```python
from build123d import *

# Parameters (mm, degrees)
F1_DEPTH = 3
F2_R     = 1.25
F3_DEPTH = 12.5
F4_R     = 1.25
F5_DEPTH = 4


# Not quite as in the source:
# - a feature names something its author has since deleted; it is built from what else it names


with BuildPart() as f1:
    # F0 (on Top) → F1 (new body, symmetric)
    with BuildSketch(Plane.XY):
        Polygon((-38.3288674057, 0), (-57, 0), (-57, -2), (0, -2), (0, 0), (-3.9376540358, 0), (-6.9237630814, 0), (-9.9603020251, 0), (-9.9603020251, 3.6380901354), (-57.4212029734, 32.3077111831), (-58.4553107619, 30.595805496), (-38.3288674057, 18.4380610677), align=None)
        Polygon((-35.6059968472, 0), (-35.6059968472, 17.1079821885), (-12.5451418841, 3.3529622977), (-12.5451418841, 0), align=None, mode=Mode.SUBTRACT)
    extrude(amount=F1_DEPTH, both=True)

    # F2 (on face) → F3 (cut, symmetric)
    with BuildSketch(Plane.XZ.offset(2)):
        with Locations((-53, 0)):
            Circle(F2_R)
        with Locations((-4, 0)):
            Circle(F2_R)
    extrude(amount=F3_DEPTH, both=True, mode=Mode.SUBTRACT)

    # F4 (on face) → F5 (cut)
    with BuildSketch(Plane(origin=(-1.0527110533, -1.7427023171, 0), x_dir=(-0.8559528436, 0.5170538943, 0), z_dir=(0.5170538943, 0.8559528436, 0))):
        with Locations((63.8546698487, 0)):
            Circle(F4_R)
        with Locations((14.8546698487, 0)):
            Circle(F4_R)
    extrude(amount=-F5_DEPTH, mode=Mode.SUBTRACT)


solid = f1.part
```
Source: CAD feature listing. Evaluate the final solid. Frame: model axes, mm. A direction names the side the tool comes from. Coordinates: 2 decimals unless noted, no trailing zeros. Loops run counter-clockwise (first coordinate to the right, second up) from the corner with the lowest first, then second, coordinate; pieces in that order, holes last. Notation, with made-up numbers: M 16.25,44.5 L 28.25,44.5 A16 cw 28.25,62.5 Z; hole C 42,-17.75 d7. An arc over 180 degrees is marked long. Put each result on its own line as item: value. Start each with the question number.
1) Contact query for flat-ended pins moving along their axis: pin 1 Ø3 at (x, z) = (-26, -0.5) entering from +Y; pin 2 Ø1.6 at (y, z) = (-1.5, 0.5) entering from -X; pin 3 Ø3 at (y, z) = (2, 0.5) entering from +X; pin 4 Ø1.5 at (x, y) = (-13.5, 6) entering from +Z. Output: stop coordinate, or through.
2) Cut plane C-C on y = 7.5. Return the cut outline in (x, z), then the cut area to 3 significant figures.
3) Pull-direction query (X, two-part tool) for faces 4 (the face through (0, -1, 0)), 5 (the face through (-57.931, 31.464, 0.042)), 6 (the face through (-48, 0, 0)), 7 (the face through (-35.606, 8, 0)); classes: pulls with the +X half, pulls with the -X half, needs draft (parallel to the pull), parting line crosses it, or undercut.
4) Cut plane B-B on z = 2.4. Return the cut outline in (x, y).
5) Reachability of faces 1 (the face through (-12.545, 2, 0)), 2 (the face through (-48.53, 24.6, 0.04)), 3 (the face through (-51.81, -1.01, 0.38)) from +Z, -Z, +X, -X, +Y, -Y: full face, straight path, thin tool, end or side. Return the list, or none.
6) Cut plane A-A on x = -4. Return the cut outline in (y, z).
7) Cut plane D-D on x = -53. Return the cut outline in (y, z).
8) Ray query, L1, parallel to X at y = 1.5, z = -2.4; L2, parallel to Z at x = -53, y = -1.2; L3, parallel to Y at x = -18.5, z = 1.25. Return the intervals inside material, ascending. Write a range as from..to.
The answers:
1. pin 1: stops at y = 14.23
1. pin 2: stops at x = -57
1. pin 3: stops at x = -9.96
1. pin 4: stops at z = 3
2. outline: M -38.33,-3 L -35.61,-3 L -35.61,3 L -38.33,3 Z; M -19.5,-3 L -16.35,-3 L -16.35,3 L -19.5,3 Z
2. area: 35.2 mm²
3. face 4: pulls with the +X half
3. face 5: pulls with the -X half
3. face 6: needs draft
3. face 7: undercut
4. outline: M -58.46,30.6 L -38.33,18.44 L -38.33,0 L -57,0 L -57,-2 L 0,-2 L 0,0 L -9.96,0 L -9.96,3.64 L -57.42,32.31 Z; hole M -35.61,0 L -12.55,0 L -12.55,3.35 L -35.61,17.11 Z
5. face 1: +Z, -Z
5. face 2: +Z, -Z, -X
5. face 3: -Y
6. outline: M -2,-3 L 0,-3 L 0,-1.25 L -2,-1.25 Z; M -2,1.25 L 0,1.25 L 0,3 L -2,3 Z
7. outline: M -2,-3 L 0,-3 L 0,-1.25 L -2,-1.25 Z; M -2,1.25 L 0,1.25 L 0,3 L -2,3 Z; M 27.3,-3 L 29.64,-3 L 29.64,3 L 27.3,3 Z
8. L1: x = -38.33..-35.61, -12.55..-9.96
8. L2: z = -3..-1.25, 1.25..3
8. L3: y = -2..0, 6.9..8.8
